Can you work these out from the model? Positions are in its coordinate system, mm. Face numbers are marked on the shaded views. A direction names the side the tool comes from. Give positions to 0.01 mm unless a question says otherwise; leave off trailing zeros. Write each loop counter-clockwise with the first axis right and the second up, starting at its lowest first coordinate (ties: lowest second). Pieces come first, ordered by that corner, then holes. Notation, with made-up numbers: (56, 39) - (104, 39) arc R16 cw to (104, 67) - close; hole circle Ø5 at (56, 53.5). An arc over 180 degrees is marked (long way). Return JSON: item names as keys, results as strings. Group by question number.
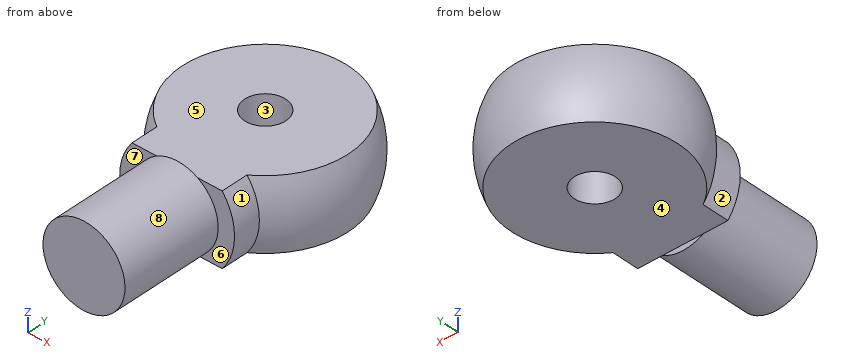
from build123d import *

# Parameters (mm, degrees)
SKETCH1_R               = 7.62
BOSS_EXTRUDE1_DEPTH     = 19.05
CUT_EXTRUDE1_DEPTH      = 59.815433775
CUT_EXTRUDE1_DEPTH_BACK = 59.815433775
SKETCH3_W               = 21.634870399
SKETCH3_H               = 44.538154166
SKETCH3_W_2             = 24.953070172
CUT_EXTRUDE2_DEPTH      = 59.142460648
CUT_EXTRUDE2_DEPTH_BACK = 59.142460648
SKETCH4_R               = 3.81


with BuildPart() as part:
    # Sketch1 → Boss-Extrude1 (new body)
    with BuildSketch(Plane(origin=(0, 0, 0), x_dir=(1, 0, 0), z_dir=(0, 1, 0))):
        with Locations(Location((0, 0, 0), (0, 0, 270))):
            Circle(SKETCH1_R)
    extrude(amount=BOSS_EXTRUDE1_DEPTH)

    # Sketch2 → Revolve1 (revolve)
    with BuildSketch(Plane(origin=(0, 0, 0), x_dir=(0, 0, -1), z_dir=(1, 0, 0)), mode=Mode.PRIVATE) as revolve1_sk:
        with BuildLine():
            Line((-10.668, 19.05), (-10.668, 24.13))
            ThreePointArc((-10.668, 24.13), (-15.776826607, 42.729323061), (0, 53.825568814))
            Line((0, 53.825568814), (0, 19.05))
            Line((0, 19.05), (-10.668, 19.05))
        make_face()
    revolve(revolve1_sk.sketch.rotate(Axis((0, 19.05, 0), (0, 1, 0)), 180), axis=Axis((0, 19.05, 0), (0, 1, 0)))

    # Sketch3 → Cut-Extrude1 (cut, two sides: drawn at the far end of the back side and taken through both)
    with BuildSketch(Plane(origin=(0, 0, 0), x_dir=(0, 0, -1), z_dir=(1, 0, 0)).offset(-CUT_EXTRUDE1_DEPTH_BACK)):
        with Locations((-17.4214352, 41.319077083)):
            Rectangle(SKETCH3_W, SKETCH3_H)
        with Locations((19.080535086, 41.319077083)):
            Rectangle(SKETCH3_W_2, SKETCH3_H)
    extrude(amount=CUT_EXTRUDE1_DEPTH + CUT_EXTRUDE1_DEPTH_BACK, mode=Mode.SUBTRACT)

    # Sketch4 → Cut-Extrude2 (cut, two sides: drawn at the far end of the back side and taken through both)
    with BuildSketch(Plane(origin=(0, 0, -6.604), x_dir=(-1, 0, 0), z_dir=(0, 0, -1)).offset(-CUT_EXTRUDE2_DEPTH_BACK)):
        with Locations((0, 37.061568814)):
            Circle(SKETCH4_R)
    extrude(amount=CUT_EXTRUDE2_DEPTH + CUT_EXTRUDE2_DEPTH_BACK, mode=Mode.SUBTRACT)


solid = part.part
1) On a 3-axis mill with a long thin cutter (end or side, diameter ignored), from which of +Z, -Z, +X, -X, +Y, -Y can I reach the whole of each face in a straight line? I mean the marked faces 5, 6, 7 and 8. Say none if no direction works.
2) Imagine slicing it at D-D, the plane z = -3.25. Write out the boundary of the cut face in (x, y), and give its area (3 significant figures).
3) We'd pull the mould along X, two halves only. Please class the marked faces 1, 2, 3 and 4: pulls with the +X half, pulls with the -X half, needs draft (parallel to the pull), parting line crosses it, or undercut.
4) Imagine slicing it at C-C, the plane x = 9.5. Write out the boundary of the cut face in (y, z), and give its area (3 significant figures).
5) Imagine slicing it at B-B, the plane z = 6. Write out the boundary of the cut face in (x, y).
6) Will these pins go through, and if not, where does the flat tip stop? pin 1 Ø9 at (x, y) = (1, 31) entering from +Z; pin 2 Ø1.1 at (x, z) = (1.5, -7) entering from +Y; pin 3 Ø2 at (x, y) = (6.5, 7.5) entering from +Z.
7) Imagine slicing it at A-A, the plane x = 0. Write out the boundary of the cut face in (y, z), and give its area (3 significant figures).
8) I need wall thicknesses on line 1 along Z through (x, y) = (-4.5, 40.5); line 2 along Y through (x, z) = (1, 1.5); line 3 along Y through (x, z) = (-2.5, -1.25). Which ranges of each line are inside material? Lowest first, please.
Resolved:
{
 "1": {"face 5": "+Z, +X, -X, +Y", "face 6": "+X, -Y", "face 7": "-X, -Y", "face 8": "-Y"},
 "2": {"outline": "(-10.16, 19.05) - (-6.89, 19.05) - (-6.89, 0) - (6.89, 0) - (6.89, 19.05) - (10.16, 19.05) - (10.16, 24.13) arc R16.45 ccw (long way) to (-10.16, 24.13) - close; hole circle Ø7.62 at (0, 37.06)", "area": "1,120 mm^2"},
 "3": {"face 1": "pulls with the +X half", "face 2": "pulls with the -X half", "face 3": "undercut", "face 4": "needs draft"},
 "4": {"outline": "(19.05, -4.85) - (24.13, -4.85) arc R13.81 ccw to (24.93, -6.6) - (49.19, -6.6) arc R13.81 ccw to (49.19, 6.6) - (24.93, 6.6) arc R13.81 ccw to (24.13, 4.85) - (19.05, 4.85) - close", "area": "394 mm^2"},
 "5": {"outline": "(-8.82, 19.05) - (-4.7, 19.05) - (-4.7, 0) - (4.7, 0) - (4.7, 19.05) - (8.82, 19.05) - (8.82, 24.13) arc R15.65 ccw (long way) to (-8.82, 24.13) - close; hole circle Ø7.62 at (0, 37.06)"},
 "6": {"pin 1": "z = 6.6", "pin 2": "y = 52.47", "pin 3": "z = 5.27"},
 "7": {"outline": "(0, -7.62) - (19.05, -7.62) - (19.05, -6.6) - (33.25, -6.6) - (33.25, 6.6) - (19.05, 6.6) - (19.05, 7.62) - (0, 7.62) - close; (40.87, -6.6) - (52.47, -6.6) arc R16.76 ccw to (52.47, 6.6) - (40.87, 6.6) - close", "area": "643 mm^2"},
 "8": {"line 1": "-6.6 to 6.6", "line 2": "0 to 33.39, 40.74 to 53.73", "line 3": "0 to 34.19, 39.94 to 53.59"}
}
